Build history of the part. All positions in model axes, mm. Give positions to 0.01 mm unless a question says otherwise; leave off trailing zeros. Write each loop counter-clockwise with the first axis right and the second up, starting at its lowest first coordinate (ties: lowest second). Pieces come first, ordered by that corner, then holes. Notation, with made-up numbers: M 2.25,60 L 15.25,60 A21 ccw 15.25,91 Z; hole C 74,59.5 d6. An arc over 180 degrees is marked long. Return JSON: item names as keys, results as strings. Group by question number.
Q1. Flat gauge pins, fed straight in: pin 1 Ø8 at (x, z) = (109.5, -1) entering from -Y; pin 2 Ø4 at (x, z) = (172, -6.5) entering from -Y. Where does each tip first touch, or does it go through?
Q2. Band-saw the part on D-D, the plane z = -30. Give the cut face in (x, y), then the cut area to 3 significant figures.
Q3. Wall check: probe 1 along X at (y, z) = (-43, -5); probe 2 along Z at (x, y) = (13, -4); probe 3 along Y at (x, z) = (121, 4.5). Give the ranges that are in metal, low to high.
Q4. Band-saw the part on B-B, the plane z = 0. Give the cut face in (x, y), then the cut area to 3 significant figures.
Q5. Pull direction X, two halves, no side cores. Call faces 1 (the cylindrical face through (0.99, -59.94, 2.64)), 2 (the cylindrical face through (100.6, -7.493, 0.33)), 3 (the flat face through (204, -1, 1)): +X half, -X half, draft (parallel to the pull), parting line (faces both ways), or undercut.
Q6. Band-saw the part on A-A, the plane y = 46. Give the cut face in (x, z), then the cut area to 3 significant figures.
from build123d import *

# Parameters (mm, degrees)
F0_R     = 60
F0_R_2   = 7.5
F1_DEPTH = 2
F2_R     = 7.5
F3_DEPTH = 200
F5_R     = 60
F6_DEPTH = 2


with BuildPart() as f1:
    # F0 (on Right) → F1 (new body)
    with BuildSketch(Plane.YZ):
        Circle(F0_R)
        Circle(F0_R_2, mode=Mode.SUBTRACT)
        Circle(F0_R_2)
    extrude(amount=F1_DEPTH)

    # F2 (on face) → F3 (join)
    with BuildSketch(Plane.YZ.offset(2)):
        Circle(F2_R)
    extrude(amount=F3_DEPTH)

    # F5 (on face) → F6 (join)
    with BuildSketch(Plane.YZ.offset(202)):
        Circle(F5_R)
    extrude(amount=F6_DEPTH)


solid = f1.part
From the geometry:
{
 "1": {"pin 1": "stops at y = -7.5", "pin 2": "stops at y = -6"},
 "2": {"outline": "M 0,-51.96 L 2,-51.96 L 2,51.96 L 0,51.96 Z; M 202,-51.96 L 204,-51.96 L 204,51.96 L 202,51.96 Z", "area": "416 mm^2"},
 "3": {"probe 1": "x = 0 to 2, 202 to 204", "probe 2": "z = -6.34 to 6.34", "probe 3": "y = -6 to 6"},
 "4": {"outline": "M 0,-60 L 2,-60 L 2,-7.5 L 202,-7.5 L 202,-60 L 204,-60 L 204,60 L 202,60 L 202,7.5 L 2,7.5 L 2,60 L 0,60 Z", "area": "3,480 mm^2"},
 "5": {"face 1": "draft", "face 2": "undercut", "face 3": "+X half"},
 "6": {"outline": "M 0,-38.52 L 2,-38.52 L 2,38.52 L 0,38.52 Z; M 202,-38.52 L 204,-38.52 L 204,38.52 L 202,38.52 Z", "area": "308 mm^2"}
}
